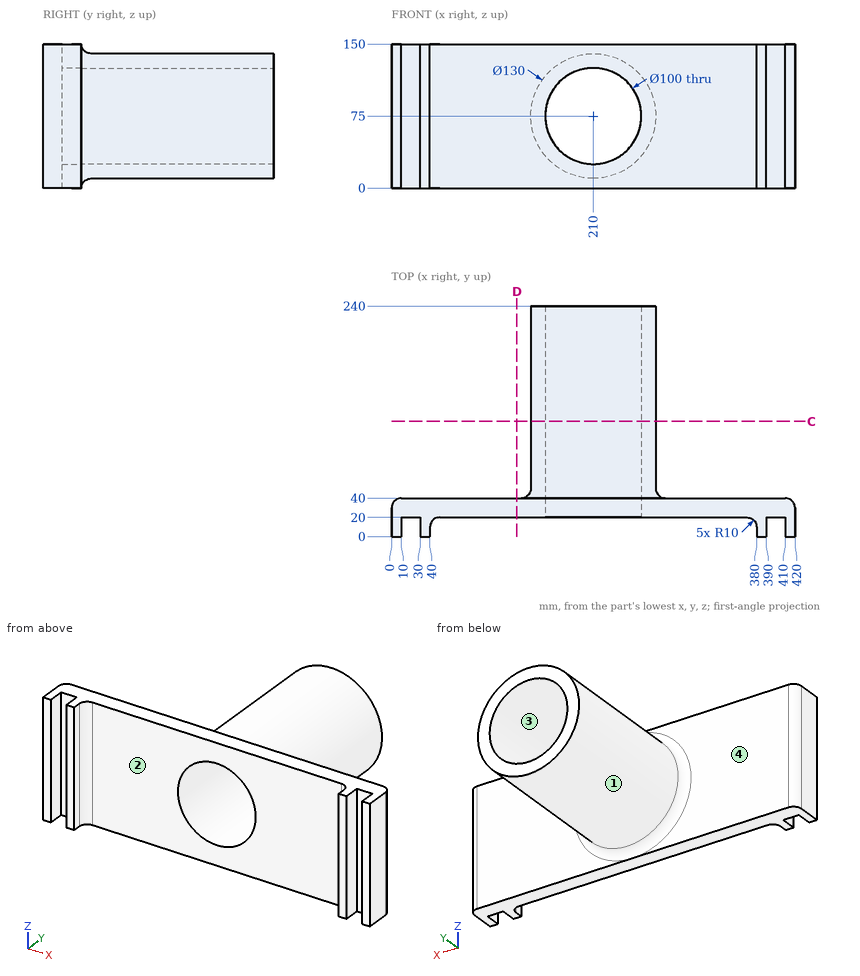
Print and shaded views of the part. All mm, measured from the part's lowest x, y and z. Round coordinates to 2 decimals unless told otherwise and drop trailing zeros. Write each loop counter-clockwise with the first axis right and the second up, starting at its lowest first coordinate (ties: lowest second). Pieces come first, ordered by that corner, then holes. Notation, with made-up numbers: M 3.25,-16.75 L 56.25,-16.75 A12 ccw 56.25,-9.75 Z; hole C -28.75,80 d9. An arc over 180 degrees is marked long. Use a Markdown table: item, result. Add a question column.
1. Slice it at C-C on y = 120. Give the cut face in (x, z), then the cut area to 3 significant figures.
2. Drill centre lines: probe 1 along Y at (x, z) = (368, 7.5); probe 2 along Z at (x, y) = (212, 73.5); probe 3 along X at (y, z) = (64, 48.5). Where is each one in solid material? Low to high.
3. Flat gauge pins, fed straight in: P1, Ø3, axis at x = 67.5, z = 95.5, coming from the -Y side; P2, Ø5, axis at x = 161, y = 110.5, coming from the +Z side; P3, Ø3, axis at y = 202.5, z = 73.5, coming from the -X side. Where does each tip first touch, or does it go through?
4. Slice it at D-D on x = 130.5. Give the cut face in (y, z), then the cut area to 3 significant figures.
5. Pull direction X, two halves, no side cores. Call the marked faces 1, 2, 3 and 4: released by +X, released by -X, zero draft, split by the parting line, or undercut.
Reply:
| question | item | result |
|---|---|---|
| 1 | outline | C 210,75 d130; hole C 210,75 d100 |
| 1 | area | 5,420 mm^2 |
| 2 | probe 1 | y = 20 to 40 |
| 2 | probe 2 | z = 10.03 to 25.04, 124.96 to 139.97 |
| 2 | probe 3 | x = 150.65 to 167.6, 252.4 to 269.35 |
| 3 | P1 | stops at y = 20 |
| 3 | P2 | stops at z = 120.42 |
| 3 | P3 | stops at x = 145 |
| 4 | outline | M 20,0 L 40,0 L 40,150 L 20,150 Z |
| 4 | area | 3,000 mm^2 |
| 5 | face 1 | split by the parting line |
| 5 | face 2 | undercut |
| 5 | face 3 | undercut |
| 5 | face 4 | zero draft |
